Geometry: final body of the model. Coordinates: model frame, mm. Face numbers are marked on the shaded views. Give positions to 0.01 mm unless a question says otherwise; leave off trailing zeros. Loops run counter-clockwise (first coordinate to the right, second up) from the corner with the lowest first, then second, coordinate; pieces in that order, holes last. Notation, with made-up numbers: (-34, 43.5) -> (-20, 43.5) arc R8 ccw to (-20, 54.5) -> close; hole circle Ø8 at (73.25, 37). An arc over 180 degrees is marked (long way). One line per item, written item: value. Start each with the question number.
from build123d import *

# Parameters (mm, degrees)
CYLINDER_R               = 11.5
CYLINDER_DEPTH           = 8.8
PRISM001_DEPTH           = 16
CUBE002_W                = 5
CUBE002_H                = 10
CUBE002_DEPTH            = 4.2
UNION001_PLACEMENT_ANGLE = 135
PRISM002_DEPTH           = 16
CUBE003_W                = 5
CUBE003_H                = 10
CUBE003_DEPTH            = 4.2
UNION002_PLACEMENT_ANGLE = 225.000007
PRISM003_DEPTH           = 16
CUBE004_W                = 5
CUBE004_H                = 10
CUBE004_DEPTH            = 4.2
UNION003_PLACEMENT_ANGLE = -45
PRISM_DEPTH              = 16
CUBE001_W                = 5
CUBE001_H                = 10
CUBE001_DEPTH            = 4.2
UNION_PLACEMENT_ANGLE    = 45
CUBE_W                   = 42
CUBE_H                   = 42
CUBE_DEPTH               = 4


with BuildPart() as cylinder:
    # cylinder → cylinder (new body)
    with BuildSketch(Plane.XY.offset(-4.4)):
        Circle(CYLINDER_R)
    extrude(amount=CYLINDER_DEPTH)


with BuildPart() as prism001:
    # prism001 → prism001 (new body)
    with BuildSketch(Plane(origin=(21.9203, 0, -8), x_dir=(1, 0, 0), z_dir=(0, 0, 1))):
        Polygon((1.6, 0), (1.385641, 0.8), (0.8, 1.385641), (0, 1.6), (-0.8, 1.385641), (-1.385641, 0.8), (-1.6, 0), (-1.385641, -0.8), (-0.8, -1.385641), (0, -1.6), (0.8, -1.385641), (1.385641, -0.8), align=None)
    extrude(amount=PRISM001_DEPTH)


with BuildPart() as union001:
    # cube002 → cube002 (new body)
    with BuildSketch(Plane(origin=(25.8345, -5, -0.1), x_dir=(1, 0, 0), z_dir=(0, 0, 1))):
        with Locations((2.5, 5)):
            Rectangle(CUBE002_W, CUBE002_H)
    extrude(amount=CUBE002_DEPTH)

    # union001: union prism001
    add(prism001.part)


with BuildPart() as union001_1:
    # union001 placement: moved
    add(union001.part.rotate(Axis((0, 0, 0), (0, 0, 1)), UNION001_PLACEMENT_ANGLE))


with BuildPart() as prism002:
    # prism002 → prism002 (new body)
    with BuildSketch(Plane(origin=(21.9203, 0, -8), x_dir=(1, 0, 0), z_dir=(0, 0, 1))):
        Polygon((1.6, 0), (1.385641, 0.8), (0.8, 1.385641), (0, 1.6), (-0.8, 1.385641), (-1.385641, 0.8), (-1.6, 0), (-1.385641, -0.8), (-0.8, -1.385641), (0, -1.6), (0.8, -1.385641), (1.385641, -0.8), align=None)
    extrude(amount=PRISM002_DEPTH)


with BuildPart() as union002:
    # cube003 → cube003 (new body)
    with BuildSketch(Plane(origin=(25.8345, -5, -0.1), x_dir=(1, 0, 0), z_dir=(0, 0, 1))):
        with Locations((2.5, 5)):
            Rectangle(CUBE003_W, CUBE003_H)
    extrude(amount=CUBE003_DEPTH)

    # union002: union prism002
    add(prism002.part)


with BuildPart() as union002_1:
    # union002 placement: moved
    add(union002.part.rotate(Axis((0, 0, 0), (0, 0, 1)), UNION002_PLACEMENT_ANGLE))


with BuildPart() as prism003:
    # prism003 → prism003 (new body)
    with BuildSketch(Plane(origin=(21.9203, 0, -8), x_dir=(1, 0, 0), z_dir=(0, 0, 1))):
        Polygon((1.6, 0), (1.385641, 0.8), (0.8, 1.385641), (0, 1.6), (-0.8, 1.385641), (-1.385641, 0.8), (-1.6, 0), (-1.385641, -0.8), (-0.8, -1.385641), (0, -1.6), (0.8, -1.385641), (1.385641, -0.8), align=None)
    extrude(amount=PRISM003_DEPTH)


with BuildPart() as union003:
    # cube004 → cube004 (new body)
    with BuildSketch(Plane(origin=(25.8345, -5, -0.1), x_dir=(1, 0, 0), z_dir=(0, 0, 1))):
        with Locations((2.5, 5)):
            Rectangle(CUBE004_W, CUBE004_H)
    extrude(amount=CUBE004_DEPTH)

    # union003: union prism003
    add(prism003.part)


with BuildPart() as union003_1:
    # union003 placement: moved
    add(union003.part.rotate(Axis((0, 0, 0), (0, 0, 1)), UNION003_PLACEMENT_ANGLE))


with BuildPart() as prism:
    # prism → prism (new body)
    with BuildSketch(Plane(origin=(21.9203, 0, -8), x_dir=(1, 0, 0), z_dir=(0, 0, 1))):
        Polygon((1.6, 0), (1.385641, 0.8), (0.8, 1.385641), (0, 1.6), (-0.8, 1.385641), (-1.385641, 0.8), (-1.6, 0), (-1.385641, -0.8), (-0.8, -1.385641), (0, -1.6), (0.8, -1.385641), (1.385641, -0.8), align=None)
    extrude(amount=PRISM_DEPTH)


with BuildPart() as union004:
    # cube001 → cube001 (new body)
    with BuildSketch(Plane(origin=(25.8345, -5, -0.1), x_dir=(1, 0, 0), z_dir=(0, 0, 1))):
        with Locations((2.5, 5)):
            Rectangle(CUBE001_W, CUBE001_H)
    extrude(amount=CUBE001_DEPTH)

    # union: union prism
    add(prism.part)


with BuildPart() as union004_1:
    # union placement: moved
    add(union004.part.rotate(Axis((0, 0, 0), (0, 0, 1)), UNION_PLACEMENT_ANGLE))

    # Group: union union001, union002, union003
    add(union001_1.part)
    add(union002_1.part)
    add(union003_1.part)

    # union004: union cylinder
    add(cylinder.part)


with BuildPart() as difference:
    # cube → cube (new body)
    with BuildSketch(Plane(origin=(-21, -21, 0), x_dir=(1, 0, 0), z_dir=(0, 0, 1))):
        with Locations((21, 21)):
            Rectangle(CUBE_W, CUBE_H)
    extrude(amount=CUBE_DEPTH)

    # difference: cut union004
    add(union004_1.part, mode=Mode.SUBTRACT)


solid = difference.part
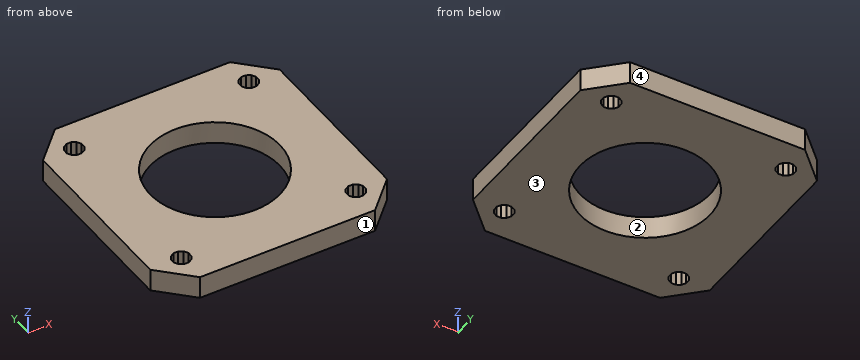
Item 1: Section C-C, the plane z = 0.7. State how many separate pieces and enclosed holes the cut face has, then the cut area to 3 significant figures.
Item 2: Section A-A, the plane x = 0. Output: boundary loops of the cut face in (y, z), then the cut area to 3 significant figures.
Item 3: Mould query, pull axis Y, two halves, no side actions, for the marked faces 1, 2, 3 and 4. Classes: pulls with the +Y half, pulls with the -Y half, needs draft (parallel to the pull), parting line crosses it, or undercut.
Item 4: Ray query, line 1 along X through (y, z) = (0, 3.25); line 2 along Y through (x, z) = (15.5, 3.85). Return the intervals inside material, ascending. Write a range as [from, to].
Geometry check:
1. separate pieces: 1
1. enclosed holes: 5
1. area: 1,260 mm2
2. outline: (-21, 0) -> (-11.5, 0) -> (-11.5, 4) -> (-21, 4) -> close; (11.5, 0) -> (21, 0) -> (21, 4) -> (11.5, 4) -> close
2. area: 76.0 mm2
3. face 1: pulls with the -Y half
3. face 2: undercut
3. face 3: needs draft
3. face 4: pulls with the +Y half
4. line 1: x = [-21, -11.5], [11.5, 21]
4. line 2: y = [-21, -17.05], [-13.95, 13.95], [17.05, 21]
